Read the model definition and answer for the solid it produces. Units are mm, in the model's axes. A direction names the side the tool comes from. Coordinates: 2 decimals unless noted, no trailing zeros. Loops run counter-clockwise (first coordinate to the right, second up) from the corner with the lowest first, then second, coordinate; pieces in that order, holes last.
from build123d import *

# Parameters (mm, degrees)
SKETCH1_R           = 12.25
BOSS_EXTRUDE1_DEPTH = 2.6
CUT_EXTRUDE1_REACH  = 19.518
SKETCH2_R           = 3.175
SKETCH2_R_2         = 1
SKETCH3_R           = 2.1
CUT_EXTRUDE2_DEPTH  = 1.75


with BuildPart() as part:
    # Sketch1 → Boss-Extrude1 (new body)
    with BuildSketch(Plane(origin=(0, 0, 0), x_dir=(1, 0, 0), z_dir=(0, 1, 0))):
        with Locations(Location((0, 0, 0), (0, 0, 270))):
            Circle(SKETCH1_R)
    extrude(amount=BOSS_EXTRUDE1_DEPTH)

    # Sketch2 → Cut-Extrude1 (cut, up to next)
    with BuildSketch(Plane.XZ, mode=Mode.PRIVATE) as cut_extrude1_sk1:
        with Locations(Location((0, 0, 0), (0, 0, 270))):
            Circle(SKETCH2_R)
    cut_extrude1_tool1 = extrude(cut_extrude1_sk1.sketch, amount=-CUT_EXTRUDE1_REACH, mode=Mode.PRIVATE) & part.part
    # Sketch2 → Cut-Extrude1 (cut, up to next)
    with BuildSketch(Plane.XZ, mode=Mode.PRIVATE) as cut_extrude1_sk2:
        with Locations(Location((0, 8.5, 0), (0, 0, 270))):
            Circle(SKETCH2_R_2)
    cut_extrude1_tool2 = extrude(cut_extrude1_sk2.sketch, amount=-CUT_EXTRUDE1_REACH, mode=Mode.PRIVATE) & part.part
    # Sketch2 → Cut-Extrude1 (cut, up to next)
    with BuildSketch(Plane.XZ, mode=Mode.PRIVATE) as cut_extrude1_sk3:
        with Locations(Location((0, -8.5, 0), (0, 0, 270))):
            Circle(SKETCH2_R_2)
    cut_extrude1_tool3 = extrude(cut_extrude1_sk3.sketch, amount=-CUT_EXTRUDE1_REACH, mode=Mode.PRIVATE) & part.part
    # Sketch2 → Cut-Extrude1 (cut, up to next)
    with BuildSketch(Plane.XZ, mode=Mode.PRIVATE) as cut_extrude1_sk4:
        with Locations(Location((-5.75, 0, 0), (0, 0, 270))):
            Circle(SKETCH2_R_2)
    cut_extrude1_tool4 = extrude(cut_extrude1_sk4.sketch, amount=-CUT_EXTRUDE1_REACH, mode=Mode.PRIVATE) & part.part
    # Sketch2 → Cut-Extrude1 (cut, up to next)
    with BuildSketch(Plane.XZ, mode=Mode.PRIVATE) as cut_extrude1_sk5:
        with Locations(Location((5.75, 0, 0), (0, 0, 270))):
            Circle(SKETCH2_R_2)
    cut_extrude1_tool5 = extrude(cut_extrude1_sk5.sketch, amount=-CUT_EXTRUDE1_REACH, mode=Mode.PRIVATE) & part.part
    add(cut_extrude1_tool1.solids().sort_by_distance((0, 0, 0))[0], mode=Mode.SUBTRACT)
    add(cut_extrude1_tool2.solids().sort_by_distance((0, 0, 8.5))[0], mode=Mode.SUBTRACT)
    add(cut_extrude1_tool3.solids().sort_by_distance((0, 0, -8.5))[0], mode=Mode.SUBTRACT)
    add(cut_extrude1_tool4.solids().sort_by_distance((-5.75, 0, 0))[0], mode=Mode.SUBTRACT)
    add(cut_extrude1_tool5.solids().sort_by_distance((5.75, 0, 0))[0], mode=Mode.SUBTRACT)

    # Sketch3 → Cut-Extrude2 (cut)
    with BuildSketch(Plane(origin=(0, 2.6, 0), x_dir=(1, 0, 0), z_dir=(0, 1, 0))):
        with Locations(Location((-5.75, 0, 0), (0, 0, 270))):
            Circle(SKETCH3_R)
        with Locations(Location((5.75, 0, 0), (0, 0, 270))):
            Circle(SKETCH3_R)
    extrude(amount=-CUT_EXTRUDE2_DEPTH, mode=Mode.SUBTRACT)


solid = part.part
Q1. A cutting plane is placed at D-D (x = -5.75). Give the vertices of the cut face in (y, z), then the cut area to 3 significant figures.
Findings below:
outline: (0, -10.82) - (2.6, -10.82) - (2.6, -2.1) - (0.85, -2.1) - (0.85, -1) - (0, -1) - close; (0, 1) - (0.85, 1) - (0.85, 2.1) - (2.6, 2.1) - (2.6, 10.82) - (0, 10.82) - close
area: 47.2 mm2
Q2. Determine the mould class of faces 1 (the face through (7.832, 1.737, -0.273)), 2 (the face through (-3, 0, 3)), 3 (the face through (3.68, 1.282, 11.684)) for opening direction X: +X half, -X half, draft (parallel to the pull), parting line (faces both ways), or undercut.
Findings below:
face 1: undercut
face 2: draft
face 3: parting line
Q3. A cutting plane is placed at A-A (x = 0). Give the vertices of the cut face in (y, z) (3 decimals).
Findings below:
outline: (0, -12.25) - (2.6, -12.25) - (2.6, -9.5) - (0, -9.5) - close; (0, -7.5) - (2.6, -7.5) - (2.6, -3.175) - (0, -3.175) - close; (0, 3.175) - (2.6, 3.175) - (2.6, 7.5) - (0, 7.5) - close; (0, 9.5) - (2.6, 9.5) - (2.6, 12.25) - (0, 12.25) - close
Q4. A cutting plane is placed at B-B (z = 0). Give the vertices of the cut face in (x, y) (3 decimals), then the cut area to 3 significant figures.
Findings below:
outline: (-12.25, 0) - (-6.75, 0) - (-6.75, 0.85) - (-7.85, 0.85) - (-7.85, 2.6) - (-12.25, 2.6) - close; (-4.75, 0) - (-3.175, 0) - (-3.175, 2.6) - (-3.65, 2.6) - (-3.65, 0.85) - (-4.75, 0.85) - close; (3.175, 0) - (4.75, 0) - (4.75, 0.85) - (3.65, 0.85) - (3.65, 2.6) - (3.175, 2.6) - close; (6.75, 0) - (12.25, 0) - (12.25, 2.6) - (7.85, 2.6) - (7.85, 0.85) - (6.75, 0.85) - close
area: 29.1 mm2
Q5. Which of the six approach directions +Z, -Z, +X, -X, +Y, -Y give full straight-line access (tool end or side, diameter ignored) to faces 4 (the face through (-7.8, 1.74, -0.46)), 5 (the face through (-0.6, 1.3, -7.7))?
Findings below:
face 4: +Y
face 5: +Y, -Y
Q6. A cutting plane is placed at C-C (z = -9). Give the vertices of the cut face in (x, y), then the cut area to 3 significant figures.
Findings below:
outline: (-8.31, 0) - (-0.87, 0) - (-0.87, 2.6) - (-8.31, 2.6) - close; (0.87, 0) - (8.31, 0) - (8.31, 2.6) - (0.87, 2.6) - close
area: 38.7 mm2
Q7. A flat-ended cylindrical pin translates along its axis: pin 1 Ø2.5 at (x, z) = (5.75, 0) entering from +Y. Find the tip coordinate at first contact, or state that the pin passes through.
Findings below:
pin 1: stops at y = 0.85
Q8. Straight lines are drawn through the part: probe 1 along X at (y, z) = (2, 0) (3 decimals); probe 2 along X at (y, z) = (0.65, 0) (3 decimals); probe 3 along Z at (x, y) = (0.5, 1.55). For each, find the intervals that lie inside material, in ascending order.
Findings below:
probe 1: x = -12.25 to -7.85, -3.65 to -3.175, 3.175 to 3.65, 7.85 to 12.25
probe 2: x = -12.25 to -6.75, -4.75 to -3.175, 3.175 to 4.75, 6.75 to 12.25
probe 3: z = -12.24 to -9.37, -7.63 to -3.14, 3.14 to 7.63, 9.37 to 12.24
